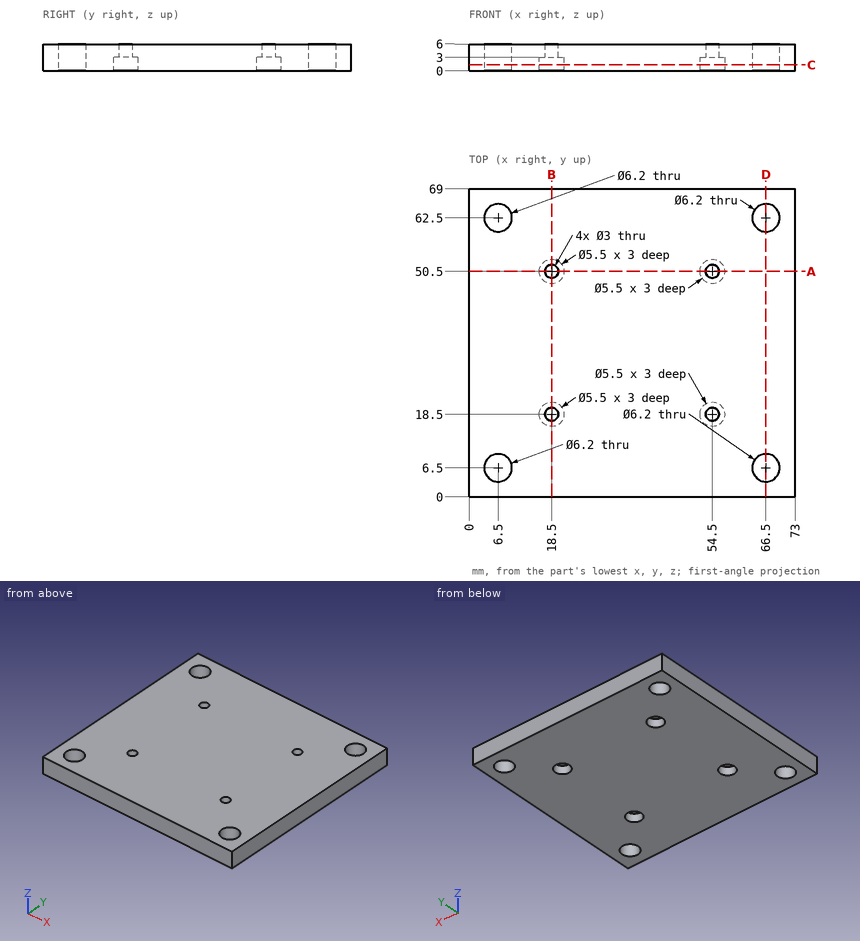
Geometry: see drawing. Coordinates: mm, zero at the bounding-box minimum. Round coordinates to 2 decimals unless told otherwise and drop trailing zeros. Order: outer loops, then holes, each group sorted by start corner. A loop starts at its lowest first (then second) coordinate and runs counter-clockwise, first axis right, second up. Notation, with made-up numbers: (75, 35) -> (111, 35) arc R21 cw to (111, 42) -> close; hole circle Ø3 at (39.25, 30.5). An arc over 180 degrees is marked (long way). Write each question's results on one line, items separated by ' | '.
Q1. Pin query (flat end, axial travel): pin 1 Ø1.6 at (x, y) = (18.5, 51.5) entering from -Z. Return the tip coordinate at first contact, or that it passes through.
Response values:
pin 1: z = 3
Q2. Section query B-B (x = 18.5). Output: boundary loops of the cut face in (y, z).
Response values:
outline: (0, 0) -> (15.75, 0) -> (15.75, 3) -> (17, 3) -> (17, 6) -> (0, 6) -> close; (20, 3) -> (21.25, 3) -> (21.25, 0) -> (47.75, 0) -> (47.75, 3) -> (49, 3) -> (49, 6) -> (20, 6) -> close; (52, 3) -> (53.25, 3) -> (53.25, 0) -> (69, 0) -> (69, 6) -> (52, 6) -> close
Q3. Ray query, line 1 along Y through (x, z) = (18.5, 2.1); line 2 along Y through (x, z) = (6.5, 4.85); line 3 along X through (y, z) = (61, 3.95). Return the intervals inside material, ascending.
Response values:
line 1: 0 to 15.75, 21.25 to 47.75, 53.25 to 69 | line 2: 0 to 3.4, 9.6 to 59.4, 65.6 to 69 | line 3: 0 to 3.79, 9.21 to 63.79, 69.21 to 73
Q4. Section query C-C (z = 1.3). Count the separate pieces of the cut face and the enclosed holes in it, and give its area (3 significant figures).
Response values:
separate pieces: 1 | enclosed holes: 8 | area: 4,820 mm²
Q5. Section query A-A (y = 50.5). Output: boundary loops of the cut face in (x, z), and give its area (3 significant figures).
Response values:
outline: (0, 0) -> (15.75, 0) -> (15.75, 3) -> (17, 3) -> (17, 6) -> (0, 6) -> close; (20, 3) -> (21.25, 3) -> (21.25, 0) -> (51.75, 0) -> (51.75, 3) -> (53, 3) -> (53, 6) -> (20, 6) -> close; (56, 3) -> (57.25, 3) -> (57.25, 0) -> (73, 0) -> (73, 6) -> (56, 6) -> close | area: 387 mm²
Q6. Section query D-D (x = 66.5). Output: boundary loops of the cut face in (y, z).
Response values:
outline: (0, 0) -> (3.4, 0) -> (3.4, 6) -> (0, 6) -> close; (9.6, 0) -> (59.4, 0) -> (59.4, 6) -> (9.6, 6) -> close; (65.6, 0) -> (69, 0) -> (69, 6) -> (65.6, 6) -> close
